```python
from build123d import *

# Parameters (mm, degrees)
F1_DEPTH = 5.08
F5_R     = 2.286
F6_DEPTH = 2.54


with BuildPart() as f1:
    # F0 (on Front) → F1 (new body)
    with BuildSketch(Plane.XZ):
        with BuildLine():
            ThreePointArc((-3.2760911955, 3.0042056319), (3.6821316631, 2.4899661475), (1.5680416715, -4.1592391512))
            Line((1.5680416715, -4.1592391512), (2.2948386219, -5.2340176442))
            ThreePointArc((2.2948386219, -5.2340176442), (4.7341692811, 3.2013850468), (-4.0028881459, 4.0789841249))
            Line((-4.0028881459, 4.0789841249), (-3.2760911955, 3.0042056319))
        make_face()
    extrude(amount=F1_DEPTH)

    # F5 (on mid) → F6 (join)
    with BuildSketch(Plane(origin=(4.2081504721, 0, 2.8456755972), x_dir=(0, 1, 0), z_dir=(0.8283760772, 0, 0.5601723617))):
        with Locations((-2.54, 0)):
            Circle(F5_R)
    extrude(amount=-F6_DEPTH)


solid = f1.part
```
Input: part model. Units: mm. Frame: model coordinates. Round coordinates to 2 decimals unless told otherwise and drop trailing zeros. Order: outer loops, then holes, each group sorted by start corner. A loop starts at its lowest first (then second) coordinate and runs counter-clockwise, first axis right, second up. Notation, with made-up numbers: (88.25, 41.25) - (136.25, 41.25) arc R20 cw to (136.25, 48.25) - close; hole circle Ø8 at (-21.5, -6). An arc over 180 degrees is marked (long way). Answer in a Markdown table with one row per item.
Item 1: Line query: line 1 (Z direction, x = 0, y = -3.7) (3 decimals); line 2 (X direction, y = -2.3, z = 0) (3 decimals); line 3 (X direction, y = -3.8, z = 0) (3 decimals). Output: solid intervals per line, ascending.
Model answer:
| item | result |
|---|---|
| line 1 | z = 4.445 to 5.715 |
| line 2 | x = 3.066 to 4.058, 4.445 to 5.715 |
| line 3 | x = 3.066 to 3.405, 4.445 to 5.715 |
Item 2: Section query A-A (y = -0.55). Return the cut outline in (x, z) (3 decimals), then the cut area to 3 significant figures.
Model answer:
| item | result |
|---|---|
| outline | (-4.003, 4.079) - (-3.276, 3.004) arc R4.445 cw to (2.932, 3.341) - (1.474, 2.355) - (2.734, 0.491) - (4.192, 1.477) arc R4.445 cw to (1.568, -4.159) - (2.295, -5.234) arc R5.715 ccw (long way) to start |
| area | 27.1 mm² |
Item 3: Section query C-C (z = -4). Return the cut outline in (x, y), then the cut area to 3 significant figures.
Model answer:
| item | result |
|---|---|
| outline | (1.94, -5.08) - (4.08, -5.08) - (4.08, 0) - (1.94, 0) - close |
| area | 10.9 mm² |
Item 4: Section query B-B (x = 0). Return the cut outline in (y, z) (3 decimals), then the cut area to 3 significant figures.
Model answer:
| item | result |
|---|---|
| outline | (-5.08, 4.445) - (0, 4.445) - (0, 5.715) - (-5.08, 5.715) - close |
| area | 6.45 mm² |
Item 5: Mould query, pull axis Z, two halves, no side actions, for faces 1 (the flat face through (4, 0, 3)), 2 (the flat face through (-3.645, -2.504, 3.549)), 3 (the cylindrical face through (2.32, -0.81, 3.79)), 4 (the flat face through (2.086, -2.572, 1.449)). Classes: released by +Z, released by -Z, zero draft, split by the parting line, or undercut.
Model answer:
| item | result |
|---|---|
| face 1 | zero draft |
| face 2 | released by -Z |
| face 3 | undercut |
| face 4 | undercut |
Item 6: Pin query (flat end, axial travel): pin 1 (2 mm diameter, centred on y = -4.5, z = 4.5, fed in from -X); pin 2 (1.5 mm diameter, centred on x = 1.5, y = -3.5, fed in from -Z); pin 3 (1 mm diameter, centred on y = -4, z = -1.5, fed in from +X); pin 4 (2 mm diameter, centred on x = -2, y = -2, fed in from +Z). Return the tip coordinate at first contact, or that it passes through.
Model answer:
| item | result |
|---|---|
| pin 1 | stops at x = -4 |
| pin 2 | stops at z = -5.17 |
| pin 3 | stops at x = 5.63 |
| pin 4 | stops at z = 5.63 |
Item 7: Section query D-D (y = -3.8). Return the cut outline in (x, z) (3 decimals).
Model answer:
| item | result |
|---|---|
| outline | (-4.003, 4.079) - (-3.276, 3.004) arc R4.445 cw to (2.257, 3.829) - (1.036, 3.003) - (3.173, -0.157) - (4.394, 0.669) arc R4.445 cw to (1.568, -4.159) - (2.295, -5.234) arc R5.715 ccw (long way) to start |
